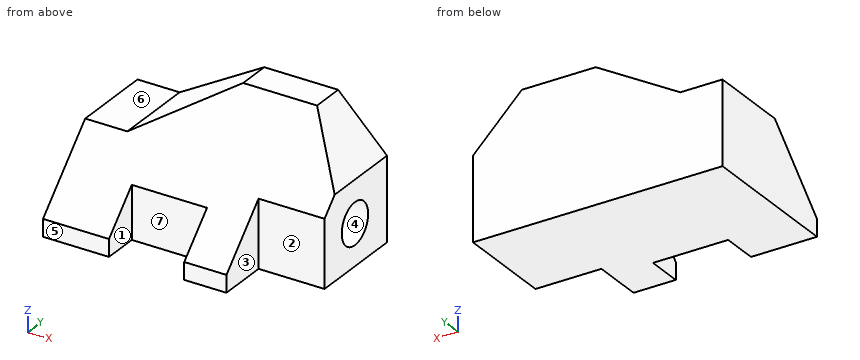
```python
from build123d import *

# Parameters (mm, degrees)
F0_W      = 96.012
F0_H      = 50.8
F1_DEPTH  = 56.896
F3_DEPTH  = 96.013
F4_W      = 28.956
F4_H      = 31.024452
F5_DEPTH  = 13.716
F6_W      = 25.4
F6_H      = 25.4
F7_DEPTH  = 19.304
F8_R      = 7.9502
F9_DEPTH  = 31.75
F11_DEPTH = 25.4
F13_DEPTH = 56.897
F15_DEPTH = 56.897


with BuildPart() as f1:
    # F0 (on Front) → F1 (new body)
    with BuildSketch(Plane.XZ):
        Rectangle(F0_W, F0_H)
    extrude(amount=F1_DEPTH)

    # F2 (on face) → F3 (cut, through all)
    with BuildSketch(Plane.YZ.offset(48.006)):
        Polygon((-56.896, -18.796), (-12.7, 25.4), (-56.896, 25.4), align=None)
    extrude(amount=-F3_DEPTH, mode=Mode.SUBTRACT)

    # F4 (on face) → F5 (cut)
    with BuildSketch(Plane.XZ.offset(56.896)):
        with Locations((-8.128, -9.887774)):
            Rectangle(F4_W, F4_H)
    extrude(amount=-F5_DEPTH, mode=Mode.SUBTRACT)

    # F6 (on face) → F7 (cut)
    with BuildSketch(Plane.XZ.offset(56.896)):
        with Locations((35.306, -12.7)):
            Rectangle(F6_W, F6_H)
    extrude(amount=-F7_DEPTH, mode=Mode.SUBTRACT)

    # F8 (on face) → F9 (cut)
    with BuildSketch(Plane.YZ.offset(48.006)):
        with Locations((-19.304, -9.652)):
            Circle(F8_R)
    extrude(amount=-F9_DEPTH, mode=Mode.SUBTRACT)

    # F10 (on face) → F11 (cut)
    with BuildSketch(Plane.YZ.offset(48.006)):
        Polygon((-38.1, 0), (-37.592, 0), (-37.592, 0.508), align=None)
    extrude(amount=-F11_DEPTH, mode=Mode.SUBTRACT)

    # F12 (on face) → F13 (cut, through all)
    with BuildSketch(Plane(origin=(0, 0, 0), x_dir=(-1, 0, 0), z_dir=(0, 1, 0))):
        Polygon((-29.21, 25.4), (-48.006, 25.4), (-48.006, 6.604), align=None)
    extrude(amount=-F13_DEPTH, mode=Mode.SUBTRACT)

    # F14 (on face) → F15 (cut, through all)
    with BuildSketch(Plane(origin=(0, 0, 0), x_dir=(-1, 0, 0), z_dir=(0, 1, 0))):
        Polygon((48.006, 25.4), (-0.762, 25.4), (31.793627, 6.604), (48.006, 6.604), align=None)
    extrude(amount=-F15_DEPTH, mode=Mode.SUBTRACT)


solid = f1.part
```
Verification items for the finished model (mm, model axes). Face numbers are marked on the shaded views. A direction names the side the tool comes from. Coordinates: 2 decimals unless noted, no trailing zeros. Write each loop counter-clockwise with the first axis right and the second up, starting at its lowest first coordinate (ties: lowest second). Pieces come first, ordered by that corner, then holes. Notation, with made-up numbers: (63.25, 18) - (97.25, 18) arc R19 cw to (97.25, 42) - close; hole circle Ø10 at (88, -18). An arc over 180 degrees is marked (long way). One line per question, with ' | ' between items. Start each with the question number.
1. Section check A-A (y = -6). Enter the section's corners in (x, z).
2. Gauge pin test, flat ends, axial feed: P1, Ø3, axis at x = -37.5, y = -48, coming from the +Z side; P2, Ø12, axis at x = -23.5, y = -30, coming from the +Z side; P3, Ø18, axis at x = -36, y = -16.5, coming from the +Z side. Record the tip position at first contact, or that the pin passes through.
3. Section check C-C (z = -8.5). Enter the section's corners in (x, y).
4. Section check B-B (x = 26). Enter the section's corners in (y, z).
5. Material ranges on line 1 along X through (y, z) = (-43.5, -18); line 2 along X through (y, z) = (-16, -4.5); line 3 along Y through (x, z) = (-18.5, -16), recorded low to high.
6. Draft check along X on the marked faces 1, 2 and 3. Enter one of: released by +X, released by -X, zero draft, split by the parting line, or undercut.
7. Section check D-D (x = 9.5). Enter the section's corners in (y, z).
8. Access from +Z, -Z, +X, -X, +Y, -Y to the whole of each face (thin tool, end or side, straight path). Record for the marked faces 4, 5, 6 and 7.
Computed values:
1) outline: (-48.01, -25.4) - (48.01, -25.4) - (48.01, 6.6) - (29.21, 25.4) - (0.76, 25.4) - (-31.79, 6.6) - (-48.01, 6.6) - close
2) P1: z = -8.4 | P2: z = 13.21 | P3: z = 9.37
3) outline: (-48.01, -46.6) - (-22.61, -46.6) - (-22.61, -43.18) - (6.35, -43.18) - (6.35, -46.6) - (22.61, -46.6) - (22.61, -37.59) - (48.01, -37.59) - (48.01, -27.17) - (16.26, -27.17) - (16.26, -11.44) - (48.01, -11.44) - (48.01, 0) - (-48.01, 0) - close
4) outline: (-37.59, -25.4) - (0, -25.4) - (0, 25.4) - (-12.7, 25.4) - (-37.59, 0.51) - close; hole circle Ø15.9 at (-19.3, -9.65)
5) line 1: -48.01 to -22.61, 6.35 to 22.61 | line 2: -48.01 to 16.26 | line 3: -43.18 to 0
6) face 1: undercut | face 2: zero draft | face 3: released by +X
7) outline: (-56.9, -25.4) - (0, -25.4) - (0, 25.4) - (-12.7, 25.4) - (-56.9, -18.8) - close
8) face 4: +X | face 5: +Z, -Z, +X, -X, -Y | face 6: +Z, -X, +Y, -Y | face 7: +Z, -Z, -Y
